Design review of the part built by this model. Coordinates are the model's own, in mm. Give positions to 0.01 mm unless a question says otherwise; leave off trailing zeros. Loops run counter-clockwise (first coordinate to the right, second up) from the corner with the lowest first, then second, coordinate; pieces in that order, holes last. Notation, with made-up numbers: (65.25, 9) - (72.25, 9) arc R21 cw to (72.25, 18) - close; hole circle Ø5 at (-14, -23). An arc over 180 degrees is marked (long way). Write each question's results on one line, items separated by ' | '.
```python
from build123d import *

# Parameters (mm, degrees)
EXTRUDE_1_DEPTH = 10


with BuildPart() as part:
    # 草图1 → 凸台-拉伸1 (new body)
    with BuildSketch(Plane.XY):
        with BuildLine():
            Line((15.08818867, 1.586238016), (15.08818867, 4.415501152))
            Line((15.08818867, 4.415501152), (-63.743519752, 4.415501152))
            Line((-63.743519752, 4.415501152), (-63.743519752, 1.586238016))
            Line((-63.743519752, 1.586238016), (-65.828448476, 1.586238016))
            Line((-65.828448476, 1.586238016), (-65.828448476, -0.512794067))
            add(Edge.make_bspline(
                [(-65.828448476, -0.512794067), (-62.716945893, -3.356182094), (-58.896356532, -5.860917235), (-54.525434698, -7.931721067)],
                knots=[5, 5, 5, 5, 6, 6, 6, 6], degree=3))
            add(Edge.make_bspline(
                [(-54.525434698, -7.931721067), (-46.10816209, -11.921636872), (-35.651823592, -14.281721066), (-24.327665541, -14.281721066)],
                knots=[6, 6, 6, 6, 7, 7, 7, 7], degree=3))
            add(Edge.make_bspline(
                [(-24.327665541, -14.281721066), (-13.00350749, -14.281721066), (-2.547168991, -11.921636872), (5.870103617, -7.931721067)],
                knots=[7, 7, 7, 7, 8, 8, 8, 8], degree=3))
            add(Edge.make_bspline(
                [(5.870103617, -7.931721067), (10.24102545, -5.860917235), (14.061614811, -3.356182094), (17.173117394, -0.512794067)],
                knots=[8, 8, 8, 8, 9, 9, 9, 9], degree=3))
            Line((17.173117394, -0.512794067), (17.173117394, 1.586238016))
            Line((17.173117394, 1.586238016), (15.08818867, 1.586238016))
        make_face()
        with BuildLine():
            add(Edge.make_bspline(
                [(-24.327665541, -5.21179665), (-25.707038709, -5.21179665), (-26.828869459, -4.093497123), (-26.828869459, -2.710614264), (-26.828869459, -1.331241095), (-25.707038709, -0.209410346), (-24.327665541, -0.209410346)],
                knots=[2, 2, 2, 2, 3, 3, 3, 4, 4, 4, 4], degree=3))
            add(Edge.make_bspline(
                [(-24.327665541, -0.209410346), (-22.948313904, -0.209410346), (-21.826483155, -1.331241095), (-21.826483155, -2.710614264), (-21.826483155, -4.093497123), (-22.948313904, -5.21179665), (-24.327665541, -5.21179665)],
                knots=[0, 0, 0, 0, 1, 1, 1, 2, 2, 2, 2], degree=3))
        make_face(mode=Mode.SUBTRACT)
    extrude(amount=EXTRUDE_1_DEPTH)


solid = part.part
```
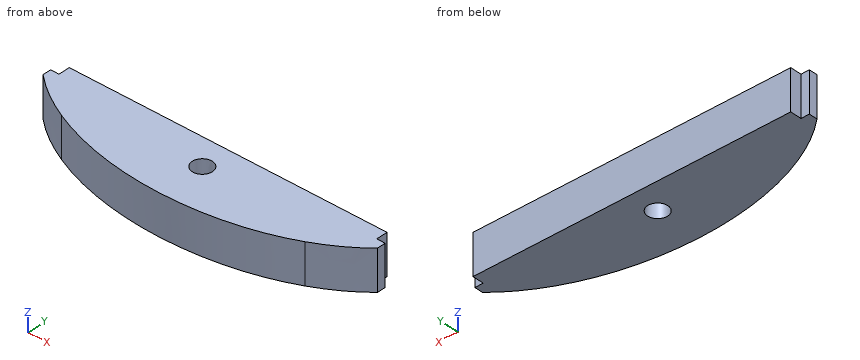
Item 1: Wall thickness on probe 1 along X at (y, z) = (-3.25, 7.5); probe 2 along Y at (x, z) = (-25.5, 6.75); probe 3 along X at (y, z) = (3, 2.75): over which ranges is each line inside the solid? List them lowest first.
Output values:
probe 1: x = -62.47 to -26.77, -21.88 to 13.82 | probe 2: y = -14.27 to -4.92, -0.5 to 4.42 | probe 3: x = -63.74 to 15.09
Item 2: We need section A-A on y = 3. Give the boundary of the cut face in (x, z), then the cut area to 3 significant figures.
Output values:
outline: (-63.74, 0) - (15.09, 0) - (15.09, 10) - (-63.74, 10) - close | area: 788 mm²
Item 3: Clearance check with flat-ended pins moving along their axes: P1, Ø1.5, axis at y = -4.5, z = 3.5, coming from the +X side; P2, Ø2, axis at x = -8.5, z = 8.5, coming from the -Y side; P3, Ø1.4, axis at y = 2.5, z = 6, coming from the -X side. State where each tip first meets the part, or that it passes through.
Output values:
P1: stops at x = 13.12 | P2: stops at y = -12.88 | P3: stops at x = -63.74
